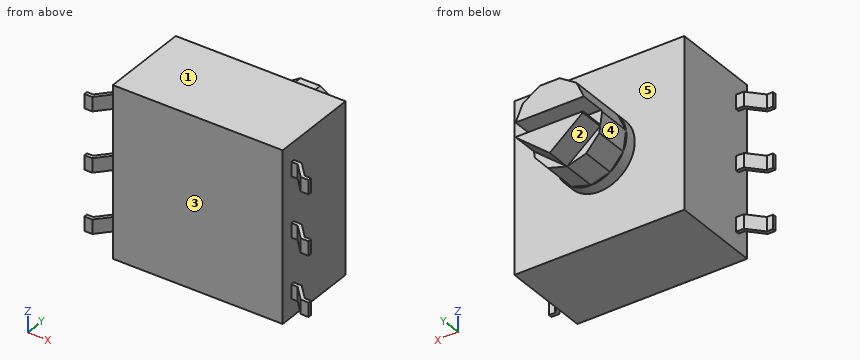
from build123d import *

# Parameters (mm, degrees)
SKETCH1_W               = 7.2
SKETCH1_H               = 7.2
BOSS_EXTRUDE1_DEPTH     = 3.8
SKETCH2_R               = 1.5
BOSS_EXTRUDE2_DEPTH     = 3
SKETCH3_R               = 1.65
CUT_EXTRUDE1_DEPTH      = 2.5
CUT_EXTRUDE2_DEPTH      = 1.05
SKETCH6_W               = 0.6
SKETCH6_H               = 0.15
LPATTERN1_COUNT         = 2
LPATTERN1_PITCH         = 2.54
LPATTERN1_COL_COUNT     = 2
LPATTERN1_COL_PITCH     = 2.54
MIRROR1_COPY_1_SKETCH_W = 0.6
MIRROR1_COPY_1_SKETCH_H = 0.15
MIRROR1_COPY_2_SKETCH_W = 0.6
MIRROR1_COPY_2_SKETCH_H = 0.15


with BuildPart() as part:
    # Sketch1 → Boss-Extrude1 (new body)
    with BuildSketch(Plane(origin=(0, 0, 0), x_dir=(1, 0, 0), z_dir=(0, 1, 0))):
        Rectangle(SKETCH1_W, SKETCH1_H)
    extrude(amount=BOSS_EXTRUDE1_DEPTH)

    # Sketch2 → Boss-Extrude2 (add)
    with BuildSketch(Plane(origin=(0, 3.8, 0), x_dir=(1, 0, 0), z_dir=(0, 1, 0))):
        Circle(SKETCH2_R)
    extrude(amount=BOSS_EXTRUDE2_DEPTH)

    # Sketch3 → Cut-Extrude1 (cut)
    with BuildSketch(Plane(origin=(0, 6.8, 0), x_dir=(1, 0, 0), z_dir=(0, 1, 0))):
        Circle(SKETCH3_R)
        Polygon((0, 1.5), (-0.810961226, 1.261880299), (-1.364447993, 0.62312252), (-1.484732163, -0.213472257), (-1.133624362, -0.982291101), (-0.422598835, -1.43923946), (0.422598835, -1.43923946), (1.133624362, -0.982291101), (1.484732163, -0.213472257), (1.364447993, 0.62312252), (0.810961226, 1.261880299), align=None, mode=Mode.SUBTRACT)
    extrude(amount=-CUT_EXTRUDE1_DEPTH, mode=Mode.SUBTRACT)

    # Sketch4 → Cut-Extrude2 (cut)
    with BuildSketch(Plane(origin=(0, 6.8, 0), x_dir=(1, 0, 0), z_dir=(0, 1, 0))):
        Polygon((1.410905998, 0.3), (-1.410905998, 0.3), (-1.484732163, -0.213472257), (-1.445216267, -0.3), (1.445216267, -0.3), (1.484732163, -0.213472257), align=None)
        Polygon((-1.364447993, 0.62312252), (-1.403086684, 0.35438452), (0, 1.5), (-0.810961226, 1.261880299), align=None)
        Polygon((0.810961226, 1.261880299), (0, 1.5), (1.403086684, 0.35438452), (1.364447993, 0.62312252), align=None)
    extrude(amount=-CUT_EXTRUDE2_DEPTH, mode=Mode.SUBTRACT)

    # Sweep1: sweep along a path in Sketch5
    with BuildLine(Plane.XY) as sweep1_path:
        Line((3.6, 0.6), (3.9, 0.6))
        Line((3.9, 0.6), (4.45, 0))
        Line((4.45, 0), (4.75, 0))
    # Sketch6 → Sweep1 (sweep)
    with BuildSketch(Plane(origin=(3.6, 0, 0), x_dir=(0, 0, -1), z_dir=(1, 0, 0))):
        with Locations((0, 0.6)):
            Rectangle(SKETCH6_W, SKETCH6_H)
    sweep1 = sweep(path=sweep1_path.line, transition=Transition.RIGHT)

    # LPattern1: Sweep1 ×2
    with Locations(*[(0, 0, -i * LPATTERN1_PITCH) for i in range(1, LPATTERN1_COUNT)]):
        add(sweep1)

    # LPattern1 col: Sweep1 ×2
    with Locations(*[(0, 0, i * LPATTERN1_COL_PITCH) for i in range(1, LPATTERN1_COL_COUNT)]):
        add(sweep1)

    # Mirror1: Sweep1 across plane
    add(sweep1.mirror(Plane(origin=(0, 0, 0), x_dir=(0, 0, 1), z_dir=(1, 0, 0))))

    # Mirror1 copy 1: sweep along a path in Mirror1 copy 1 path
    with BuildLine(Plane(origin=(0, 0, -2.54), x_dir=(-1, 0, 0), z_dir=(0, 0, 1))) as mirror1_copy_1_path:
        Line((3.6, -0.6), (3.9, -0.6))
        Line((3.9, -0.6), (4.45, 0))
        Line((4.45, 0), (4.75, 0))
    # Mirror1 copy 1 sketch → Mirror1 copy 1 (sweep)
    with BuildSketch(Plane(origin=(-3.6, 0, -2.54), x_dir=(0, 0, -1), z_dir=(-1, 0, 0))):
        with Locations((0, -0.6)):
            Rectangle(MIRROR1_COPY_1_SKETCH_W, MIRROR1_COPY_1_SKETCH_H)
    sweep(path=mirror1_copy_1_path.line, transition=Transition.RIGHT)

    # Mirror1 copy 2: sweep along a path in Mirror1 copy 2 path
    with BuildLine(Plane(origin=(0, 0, 2.54), x_dir=(-1, 0, 0), z_dir=(0, 0, 1))) as mirror1_copy_2_path:
        Line((3.6, -0.6), (3.9, -0.6))
        Line((3.9, -0.6), (4.45, 0))
        Line((4.45, 0), (4.75, 0))
    # Mirror1 copy 2 sketch → Mirror1 copy 2 (sweep)
    with BuildSketch(Plane(origin=(-3.6, 0, 2.54), x_dir=(0, 0, -1), z_dir=(-1, 0, 0))):
        with Locations((0, -0.6)):
            Rectangle(MIRROR1_COPY_2_SKETCH_W, MIRROR1_COPY_2_SKETCH_H)
    sweep(path=mirror1_copy_2_path.line, transition=Transition.RIGHT)


solid = part.part
Here's how the part is built. I have some questions about the finished solid (model axes, mm). Face numbers are marked on the shaded views. A direction names the side the tool comes from. Round coordinates to 2 decimals unless told otherwise and drop trailing zeros. Order: outer loops, then holes, each group sorted by start corner. A loop starts at its lowest first (then second) coordinate and runs counter-clockwise, first axis right, second up. Notation, with made-up numbers: (36, -20) -> (54, -20) arc R14 cw to (54, 3) -> close; hole circle Ø6 at (-27, 37.5). An arc over 180 degrees is marked (long way). Use CSV: the item, a comma, the result in double quotes.
1. I want a section at D-D on y = 3.25. List the corners of the cut face in (x, z) for me, and give its area (3 significant figures).
Recorded:
outline,"(-3.6, -3.6) -> (3.6, -3.6) -> (3.6, 3.6) -> (-3.6, 3.6) -> close"
area,"51.8 mm2"
2. Which directions (+Z, -Z, +X, -X, +Y, -Y) give clear straight access to the entire face, cutting with the end or side of a thin tool? Please do the marked faces 1 and 2.
Recorded:
face 1,"+Z, +X, -X, +Y, -Y"
face 2,"-Z, -X, +Y"
3. Thinking about a two-plate mould opening in X: for the marked faces 3, 4 and 5, which applies, pulls with the +X half, pulls with the -X half, needs draft (parallel to the pull), parting line crosses it, or undercut?
Recorded:
face 3,"undercut"
face 4,"pulls with the -X half"
face 5,"needs draft"
4. I want a section at C-C on x = -3.25. List the corners of the cut face in (y, z) for me, and give its area (3 significant figures).
Recorded:
outline,"(0, -3.6) -> (3.8, -3.6) -> (3.8, 3.6) -> (0, 3.6) -> close"
area,"27.4 mm2"
5. I want a section at A-A on y = 4.5. List the corners of the cut face in (x, z) for me, and give its area (3 significant figures).
Recorded:
outline,"(-1.48, 0.21) -> (-1.36, -0.62) -> (-0.81, -1.26) -> (0, -1.5) -> (0.81, -1.26) -> (1.36, -0.62) -> (1.48, 0.21) -> (1.13, 0.98) -> (0.42, 1.44) -> (-0.42, 1.44) -> (-1.13, 0.98) -> close"
area,"6.69 mm2"
6. I'm going to push flat-ended pins straight in: P1, Ø0.5, axis at x = -1, z = 1.5, coming from the +Y side; P2, Ø0.9, axis at x = 0, y = 5, coming from the +Z side. Where does each tip first touch, or does it pass through?
Recorded:
P1,"stops at y = 3.8"
P2,"stops at z = 1.44"
7. I need wall thicknesses on line 1 along Y through (x, z) = (-2.25, -1); line 2 along X through (y, z) = (2, 2.75); line 3 along Y through (x, z) = (-1, 0.5). Which ranges of each line are inside material? Lowest first, please.
Recorded:
line 1,"y = 0 to 3.8"
line 2,"x = -3.6 to 3.6"
line 3,"y = 0 to 6.8"
8. I want a section at B-B on z = 0. List the corners of the cut face in (x, y) for me (3 decimals).
Recorded:
outline,"(-4.75, -0.075) -> (-4.417, -0.075) -> (-3.867, 0.525) -> (-3.6, 0.525) -> (-3.6, 0) -> (3.6, 0) -> (3.6, 0.525) -> (3.867, 0.525) -> (4.417, -0.075) -> (4.75, -0.075) -> (4.75, 0.075) -> (4.483, 0.075) -> (3.933, 0.675) -> (3.6, 0.675) -> (3.6, 3.8) -> (1.5, 3.8) -> (1.5, 4.3) -> (1.454, 4.3) -> (1.454, 5.75) -> (-1.454, 5.75) -> (-1.454, 4.3) -> (-1.5, 4.3) -> (-1.5, 3.8) -> (-3.6, 3.8) -> (-3.6, 0.675) -> (-3.933, 0.675) -> (-4.483, 0.075) -> (-4.75, 0.075) -> close"
